from build123d import *

# Parameters (mm, degrees)
SKETCH1_W           = 76.2
SKETCH1_H           = 38.1
BOSS_EXTRUDE1_DEPTH = 6.35
SKETCH3_W           = 6.35
SKETCH3_H           = 5.08
BOSS_EXTRUDE2_DEPTH = 6.35
CUT_EXTRUDE1_DEPTH  = 7.35
FILLET1_R           = 6.35


with BuildPart() as part:
    # Sketch1 → Boss-Extrude1 (new body)
    with BuildSketch(Plane.XY):
        Rectangle(SKETCH1_W, SKETCH1_H)
    extrude(amount=BOSS_EXTRUDE1_DEPTH)

    # Sketch3 → Boss-Extrude2 (add)
    with BuildSketch(Plane.XY.offset(6.35)):
        with Locations((19.05, 21.59)):
            Rectangle(SKETCH3_W, SKETCH3_H)
        with Locations((-19.05, 21.59)):
            Rectangle(SKETCH3_W, SKETCH3_H)
        with Locations((0, 21.59)):
            Rectangle(SKETCH3_W, SKETCH3_H)
    extrude(amount=-BOSS_EXTRUDE2_DEPTH)

    # Sketch6 → Cut-Extrude1 (cut, through all)
    with BuildSketch(Plane.XY.offset(6.35)):
        Polygon((-11.6078, 19.05), (-11.6078, 12.7), (-13.8938, 12.7), (-13.8938, 6.7564), (-11.6078, 6.7564), (-11.6078, 3.81), (-7.4422, 3.81), (-7.4422, 6.7564), (-5.1562, 6.7564), (-5.1562, 12.7), (-7.4422, 12.7), (-7.4422, 19.05), align=None)
        Polygon((7.4422, 19.05), (7.4422, 12.7), (5.1562, 12.7), (5.1562, 6.7564), (7.4422, 6.7564), (7.4422, 3.81), (11.6078, 3.81), (11.6078, 6.7564), (13.8938, 6.7564), (13.8938, 12.7), (11.6078, 12.7), (11.6078, 19.05), align=None)
    extrude(amount=-CUT_EXTRUDE1_DEPTH, mode=Mode.SUBTRACT)

    # Fillet1
    fillet1_edges = [part.edges().sort_by_distance(p)[0] for p in [
        (38.1, -19.05, 3.175),
        (-38.1, -19.05, 3.175),
    ]]
    fillet(fillet1_edges, radius=FILLET1_R)


solid = part.part
Input: part model. Units: mm. Frame: model coordinates. A direction names the side the tool comes from. Coordinates: 2 decimals unless noted, no trailing zeros. Loops run counter-clockwise (first coordinate to the right, second up) from the corner with the lowest first, then second, coordinate; pieces in that order, holes last.
(1) First-contact query: pin 1 Ø0.7 at (x, z) = (6.5, 1.5) entering from +Y; pin 2 Ø10 at (x, y) = (6.5, 12) entering from -Z; pin 3 Ø2 at (x, z) = (-10.5, 3.5) entering from +Y; pin 4 Ø1.5 at (y, z) = (21.5, 4) entering from -X (3 decimals). Flat tips, straight axial feed; report the tip coordinate or a pass-through.
(2) Section C-C on x = 29. Return the cut outline in (y, z), then the cut area to 3 significant figures.
(3) Section A-A on y = 6. Return the cut outline in (x, z).
(4) Material intervals for probe 1 along X at (y, z) = (16.5, 3.5); probe 2 along X at (y, z) = (10, 0.5); probe 3 along Y at (x, z) = (24, 3.5), sorted ascending.
(5) Set-up query: faces 4 (the face through (-22.225, 22, 3)), 5 (the face through (-13, 6.756, 3)), 6 (the face through (-11.608, 16, 3)). Return all of +Z, -Z, +X, -X, +Y, -Y with unobstructed straight access to the full face (end or side cutting, diameter ignored); none if empty.
(6) Pull-direction query (Y, two-part tool) for faces 1 (the face through (-5, 19.05, 3)), 2 (the face through (-6, 6.756, 3)), 3 (the face through (-11.608, 5, 3)); classes: released by +Y, released by -Y, zero draft, split by the parting line, or undercut.
(7) Section B-B on y = 21. Return the cut outline in (x, z) (3 decimals).
Data:
1. pin 1: stops at y = 19.05
1. pin 2: stops at z = 0
1. pin 3: stops at y = 3.81
1. pin 4: stops at x = -22.225
2. outline: (-19.05, 0) - (19.05, 0) - (19.05, 6.35) - (-19.05, 6.35) - close
2. area: 242 mm2
3. outline: (-38.1, 0) - (-11.61, 0) - (-11.61, 6.35) - (-38.1, 6.35) - close; (-7.44, 0) - (7.44, 0) - (7.44, 6.35) - (-7.44, 6.35) - close; (11.61, 0) - (38.1, 0) - (38.1, 6.35) - (11.61, 6.35) - close
4. probe 1: x = -38.1 to -11.61, -7.44 to 7.44, 11.61 to 38.1
4. probe 2: x = -38.1 to -13.89, -5.16 to 5.16, 13.89 to 38.1
4. probe 3: y = -19.05 to 19.05
5. face 4: +Z, -Z, -X, +Y
5. face 5: +Z, -Z
5. face 6: +Z, -Z, +Y
6. face 1: released by +Y
6. face 2: undercut
6. face 3: zero draft
7. outline: (-22.225, 0) - (-15.875, 0) - (-15.875, 6.35) - (-22.225, 6.35) - close; (-3.175, 0) - (3.175, 0) - (3.175, 6.35) - (-3.175, 6.35) - close; (15.875, 0) - (22.225, 0) - (22.225, 6.35) - (15.875, 6.35) - close
